Autodesk Inventor part; units mm, degrees
ref_plane "YZ Plane" through (0, 0, 0) normal (1, 0, 0) x (0, 1, 0)
ref_plane "XZ Plane" through (0, 0, 0) normal (0, 1, 0) x (-1, 0, 0)
ref_plane "XY Plane" through (0, 0, 0) normal (0, 0, 1) x (1, 0, 0)
ref_plane "Work Plane1" through (0, 0, 0) normal (0, 0, 1) x (1, 0, 0)
sketch "Sketch1" plane through (0, 0, 0) normal (0, 0, 1) x (1, 0, 0)
  circle A0 centre (-34, 58.3124) radius 1.425
  circle A1 centre (-67.5, 0.2887) radius 1.425
  circle A2 centre (-0.5, 0.2887) radius 1.425
  arc A3 (-2.5, 3.7528) -> (-4.5, 0.2887) centre (-0.5, 0.2887) ccw
  arc A4 (-5, -0.2113) -> (-4.5, 0.2887) centre (-5, 0.2887) ccw
  line L0 (-5, -0.2113) -> (-63, -0.2113)
  arc A5 (-63.5, 0.2887) -> (-63, -0.2113) centre (-63, 0.2887) ccw
  arc A6 (-63.5, 0.2887) -> (-65.5, 3.7528) centre (-67.5, 0.2887) ccw
  arc A7 (-65.683, 4.4358) -> (-65.5, 3.7528) centre (-65.25, 4.1858) ccw
  line L1 (-65.683, 4.4358) -> (-36.683, 54.6653)
  arc A8 (-36, 54.8483) -> (-36.683, 54.6653) centre (-36.25, 54.4153) ccw
  arc A9 (-36, 54.8483) -> (-32, 54.8483) centre (-34, 58.3124) ccw
  arc A10 (-31.317, 54.6653) -> (-32, 54.8483) centre (-31.75, 54.4153) ccw
  line L2 (-31.317, 54.6653) -> (-2.317, 4.4358)
  arc A11 (-2.5, 3.7528) -> (-2.317, 4.4358) centre (-2.75, 4.1858) ccw
  line L3 (2.9641, 2.2887) -> (-30.5359, 60.3124)
  arc A12 (-30.5359, 60.3124) -> (-37.4641, 60.3124) centre (-34, 58.3124) ccw
  line L4 (-37.4641, 60.3124) -> (-70.9641, 2.2887)
  arc A13 (-70.9641, 2.2887) -> (-67.5, -3.7113) centre (-67.5, 0.2887) ccw
  line L5 (-67.5, -3.7113) -> (-0.5, -3.7113)
  arc A14 (-0.5, -3.7113) -> (2.9641, 2.2887) centre (-0.5, 0.2887) ccw
  circle A15 centre (-34, 58.3124) radius 1.45
  circle A16 centre (-0.5, 0.2887) radius 1.45
  circle A17 centre (-67.5, 0.2887) radius 1.45
  line L6 (-67.5, 0.2887) -> (-13.7859, 31.3005) construction
  line L7 (-0.5, 0.2887) -> (-54.2141, 31.3005) construction
  point P0 (0, 0)
  point P1 (-34, 19.6299)
  dimension "d0" = 2.9
extrude "Extrusion1" add sketch "Sketch1" along normal blind 3 contours A3 A4 L0 A5 A6 A7 L1 A8 A9 A10 L2 A11 | A14 L5 A13 L4 A12 L3
sketch "Sketch2" plane through (0, 0, 3) normal (0, 0, 1) x (1, 0, 0)
  line L0 (2.9641, 2.2887) -> (-30.5359, 60.3124)
  arc A0 (-30.5359, 60.3124) -> (-37.4641, 60.3124) centre (-34, 58.3124) ccw
  line L1 (-34, 58.3124) -> (-34, -3.7946) construction
  circle A1 centre (-34, 19.6299) radius 3.175
  circle A2 centre (-67.5, 0.2887) radius 1.45
  line L2 (-67.5, 0.2887) -> (-13.7859, 31.3005) construction
  circle A3 centre (-34, 27.5299) radius 1.425
  dimension "d33" = 6.35
  dimension "d34" = 2.85
  dimension "d35" = 7.9
extrude "Extrusion4" cut sketch "Sketch2" against normal through all contours A1 | A3
properties part number "ServoHousingEndPlates" material "Wood (Birch)"
Could you check a few things on this model? Use its own coordinates, in mm. Coordinates: 2 decimals unless noted, no trailing zeros. Loops run counter-clockwise (first coordinate to the right, second up) from the corner with the lowest first, then second, coordinate; pieces in that order, holes last. Notation, with made-up numbers: (83, 42.5) -> (139, 42.5) arc R28 cw to (139, 77.5) -> close; hole circle Ø1 at (19.25, 1.5). An arc over 180 degrees is marked (long way). Answer in a Markdown table with one row per item.
(1) Thinking about a two-plate mould opening in Y: for faces 1 (the face through (-34, -3.711, 1)), 2 (the face through (-68.65, 1.17, 1.48)), 3 (the face through (-13.55, 30.89, 1.48)), which applies, released by +Y, released by -Y, zero draft, split by the parting line, or undercut?
Results found:
| item | result |
|---|---|
| face 1 | released by -Y |
| face 2 | undercut |
| face 3 | released by +Y |
(2) Imagine slicing it at B-B (z = 1.55). List the corners of the cut face in (x, y) for me (3 decimals), plus the area to 3 significant figures.
Results found:
| item | result |
|---|---|
| outline | (-70.964, 2.289) arc R4 ccw to (-67.5, -3.711) -> (-0.5, -3.711) arc R4 ccw to (2.964, 2.289) -> (-30.536, 60.312) arc R4 ccw to (-37.464, 60.312) -> close; hole circle Ø2.9 at (-67.5, 0.289); hole circle Ø6.35 at (-34, 19.63); hole circle Ø2.9 at (-34, 58.312); hole circle Ø2.85 at (-34, 27.53); hole circle Ø2.9 at (-0.5, 0.289) |
| area | 2,740 mm^2 |
(3) If I drill on probe 1 along Y at (x, z) = (-34, 1); probe 2 along Y at (x, z) = (-67.5, 1.1); probe 3 along Y at (x, z) = (-1, 2.7), over which ranges is the centre line in solid material (lowest first)?
Results found:
| item | result |
|---|---|
| probe 1 | y = -3.71 to 16.45, 22.8 to 26.1, 28.95 to 56.86, 59.76 to 62.31 |
| probe 2 | y = -3.71 to -1.16, 1.74 to 8.29 |
| probe 3 | y = -3.71 to -1.07, 1.65 to 9.15 |
(4) Imagine slicing it at D-D (x = -53). List the corners of the cut face in (y, z) for me, plus the area to 3 significant figures.
Results found:
| item | result |
|---|---|
| outline | (-3.71, 0) -> (33.4, 0) -> (33.4, 3) -> (-3.71, 3) -> close |
| area | 111 mm^2 |
(5) Imagine slicing it at C-C (y = 41). List the corners of the cut face in (x, z) for me.
Results found:
| item | result |
|---|---|
| outline | (-48.61, 0) -> (-19.39, 0) -> (-19.39, 3) -> (-48.61, 3) -> close |
(6) Imagine slicing it at A-A (x = -34). List the corners of the cut face in (y, z) for me, plus the area to 3 significant figures.
Results found:
| item | result |
|---|---|
| outline | (-3.71, 0) -> (16.45, 0) -> (16.45, 3) -> (-3.71, 3) -> close; (22.8, 0) -> (26.1, 0) -> (26.1, 3) -> (22.8, 3) -> close; (28.95, 0) -> (56.86, 0) -> (56.86, 3) -> (28.95, 3) -> close; (59.76, 0) -> (62.31, 0) -> (62.31, 3) -> (59.76, 3) -> close |
| area | 162 mm^2 |
